The drawing under review shows one solid part. Ordinate dimensions are in mm from its lowest x, y, z. A direction names the side the tool comes from. Round coordinates to 2 decimals unless told otherwise and drop trailing zeros. Order: outer loops, then holes, each group sorted by start corner. A loop starts at its lowest first (then second) coordinate and runs counter-clockwise, first axis right, second up.
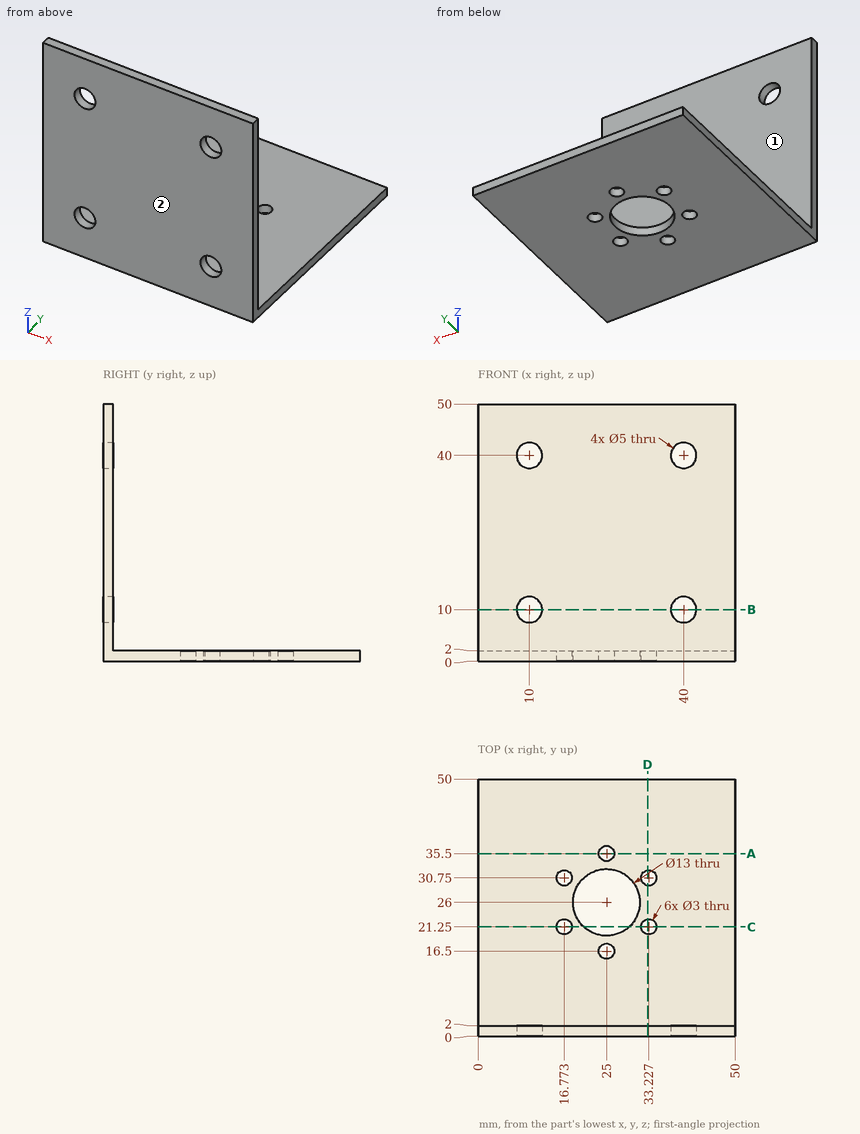
Q1. Take a section at C-C, the plane y = 21.25. State the section outline as (x, z) points.
Q2. Tool access review of the marked faces 1 and 2: name each direction out of +Z, -Z, +X, -X, +Y, -Y from which nothing blocks a thin tool from reaching the whole face with its end or side.
Q3. Wall thickness on line 1 (Y direction, x = 25, z = 1.05); line 2 (Z direction, x = 14.5, y = 24): over which ranges is each line inside the solid? List them lowest first.
Q4. Clearance check with flat-ended pins moving along their axes: pin 1 (4.5 mm diameter, centred on x = 40, z = 10, fed in from -Y); pin 2 (24 mm diameter, centred on x = 30, z = 15, fed in from +Y); pin 3 (4 mm diameter, centred on x = 33.23, y = 21.25, fed in from +Z). State where each tip first meets the part, or that it passes through.
Q5. Take a section at D-D, the plane x = 33. State the section outline as (y, z) points, plus the area to 3 significant figures.
Q6. Take a section at B-B, the plane z = 10. State the section outline as (x, y) points.
Q7. Take a section at A-A, the plane y = 35.5. State the section outline as (x, z) points.
Working result:
1. outline: (0, 0) - (15.27, 0) - (15.27, 2) - (0, 2) - close; (18.27, 0) - (20.56, 0) - (20.56, 2) - (18.27, 2) - close; (29.44, 0) - (31.73, 0) - (31.73, 2) - (29.44, 2) - close; (34.73, 0) - (50, 0) - (50, 2) - (34.73, 2) - close
2. face 1: +Z, +X, -X, +Y
2. face 2: +Z, -Z, +X, -X, -Y
3. line 1: y = 0 to 15, 18 to 19.5, 32.5 to 34, 37 to 50
3. line 2: z = 0 to 2
4. pin 1: passes through
4. pin 2: stops at y = 2
4. pin 3: stops at z = 2
5. outline: (0, 0) - (19.77, 0) - (19.77, 2) - (2, 2) - (2, 50) - (0, 50) - close; (22.73, 0) - (29.27, 0) - (29.27, 2) - (22.73, 2) - close; (32.23, 0) - (50, 0) - (50, 2) - (32.23, 2) - close
5. area: 184 mm2
6. outline: (0, 0) - (7.5, 0) - (7.5, 2) - (0, 2) - close; (12.5, 0) - (37.5, 0) - (37.5, 2) - (12.5, 2) - close; (42.5, 0) - (50, 0) - (50, 2) - (42.5, 2) - close
7. outline: (0, 0) - (23.5, 0) - (23.5, 2) - (0, 2) - close; (26.5, 0) - (50, 0) - (50, 2) - (26.5, 2) - close
